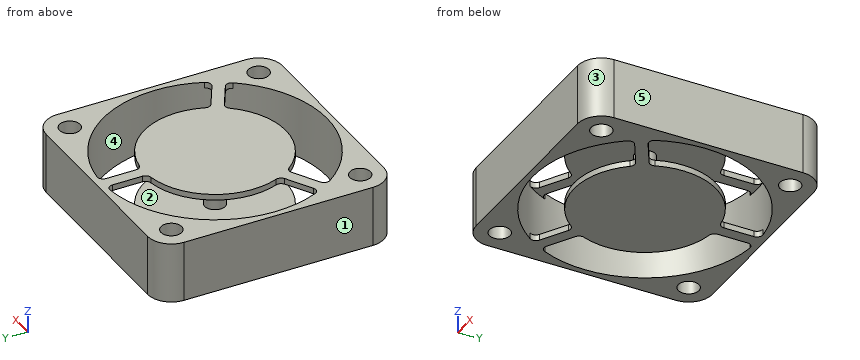
from build123d import *

# Parameters (mm, degrees)
BOSS_EXTRUDE1_DEPTH = 10.3
SKETCH2_R           = 1.75
CUT_EXTRUDE1_DEPTH  = 11.3
SKETCH3_R           = 19
SKETCH3_R_2         = 12
CUT_EXTRUDE2_DEPTH  = 11.3
BOSS_EXTRUDE2_DEPTH = 10.3
CIRPATTERN1_COUNT   = 3
FILLET2_R           = 1
CUT_EXTRUDE3_START  = 1
SKETCH5_R           = 19
CUT_EXTRUDE3_DEPTH  = 8.3
SKETCH6_R           = 1.75
BOSS_EXTRUDE3_DEPTH = 8.3


with BuildPart() as part:
    # Sketch1 → Boss-Extrude1 (new body)
    with BuildSketch(Plane.XY):
        with BuildLine():
            Line((0, -4), (32, -4))
            ThreePointArc((32, -4), (34.828427125, -2.828427125), (36, 0))
            Line((36, 0), (36, 32))
            ThreePointArc((36, 32), (34.828427125, 34.828427125), (32, 36))
            Line((32, 36), (0, 36))
            ThreePointArc((0, 36), (-2.828427125, 34.828427125), (-4, 32))
            Line((-4, 32), (-4, 0))
            ThreePointArc((-4, 0), (-2.828427125, -2.828427125), (0, -4))
        make_face()
    extrude(amount=BOSS_EXTRUDE1_DEPTH)

    # Sketch2 → Cut-Extrude1 (cut, through all)
    with BuildSketch(Plane.XY.offset(10.3)):
        Circle(SKETCH2_R)
        with Locations((0, 32)):
            Circle(SKETCH2_R)
        with Locations((32, 0)):
            Circle(SKETCH2_R)
        with Locations((32, 32)):
            Circle(SKETCH2_R)
    extrude(amount=-CUT_EXTRUDE1_DEPTH, mode=Mode.SUBTRACT)

    # Sketch3 → Cut-Extrude2 (cut, through all)
    with BuildSketch(Plane.XY.offset(10.3)):
        with Locations((16, 16)):
            Circle(SKETCH3_R)
        with Locations((16, 16)):
            Circle(SKETCH3_R_2, mode=Mode.SUBTRACT)
    extrude(amount=-CUT_EXTRUDE2_DEPTH, mode=Mode.SUBTRACT)

    # Sketch4 → Boss-Extrude2 (add)
    with BuildSketch(Plane.XY):
        with BuildLine():
            Line((15, 27.958260743), (15, 34.973665961))
            ThreePointArc((15, 34.973665961), (16, 35), (17, 34.973665961))
            Line((17, 34.973665961), (17, 27.958260743))
            ThreePointArc((17, 27.958260743), (16, 28), (15, 27.958260743))
        make_face()
    boss_extrude2 = extrude(amount=BOSS_EXTRUDE2_DEPTH)

    # CirPattern1: Boss-Extrude2 ×3 about axis
    cirpattern1_axis = Axis((16, 16, 0), (0, 0, 1))
    for i in range(1, CIRPATTERN1_COUNT):
        add(boss_extrude2.rotate(cirpattern1_axis, i * 360 / CIRPATTERN1_COUNT))

    # Fillet2
    fillet2_edges = [part.edges().sort_by_distance(p)[0] for p in [
        (15, 27.958260743, 5.15),
        (17, 27.958260743, 5.15),
        (17, 34.973665961, 5.15),
        (15, 34.973665961, 5.15),
        (6.143842411, 9.154844225, 5.15),
        (5.143842411, 10.886895032, 5.15),
        (-0.931676725, 7.379192423, 5.15),
        (0.068323275, 5.647141616, 5.15),
        (26.856157589, 10.886895032, 5.15),
        (25.856157589, 9.154844225, 5.15),
        (31.931676725, 5.647141616, 5.15),
        (32.931676725, 7.379192423, 5.15),
    ]]
    fillet(fillet2_edges, radius=FILLET2_R)

    # Sketch5 → Cut-Extrude3 (cut)
    with BuildSketch(Plane.XY.offset(CUT_EXTRUDE3_START)):
        with Locations((16, 16)):
            Circle(SKETCH5_R)
    extrude(amount=CUT_EXTRUDE3_DEPTH, mode=Mode.SUBTRACT)

    # Sketch6 → Boss-Extrude3 (add)
    with BuildSketch(Plane.XY.offset(1)):
        with Locations((16, 16)):
            Circle(SKETCH6_R)
    extrude(amount=BOSS_EXTRUDE3_DEPTH)


solid = part.part
Geometry check sheet. Reference: the model listing, model coordinates, mm. Face numbers are marked on the shaded views. A direction names the side the tool comes from. Give positions to 0.01 mm unless a question says otherwise; leave off trailing zeros. Write each loop counter-clockwise with the first axis right and the second up, starting at its lowest first coordinate (ties: lowest second). Pieces come first, ordered by that corner, then holes. Notation, with made-up numbers: M -19,53.25 L 16,53.25 A19 cw 16,73.25 Z; hole C -34,-38.75 d5. An arc over 180 degrees is marked long. Answer as CSV lines item,"result". Start each with the question number.
Q1. Section check C-C, the plane y = 19.5. Record the cut outline in (x, z), then the cut area to 3 significant figures.
Q2. Section check A-A, the plane x = 16. Record the cut outline in (y, z).
Q3. Section check D-D, the plane x = 28.5. Record the cut outline in (y, z).
Q4. Section check B-B, the plane z = 3.5. Record the cut outline in (x, y), then the cut area to 3 significant figures.
Q5. Tool access check on the marked faces 1 and 2. Record the directions out of +Z, -Z, +X, -X, +Y, -Y that give a thin tool (end or side, any length) a straight path to the whole face; none if there is none.
Q6. Release check for a two-part mould opening along Y. For the marked faces 3, 4 and 5 record: pulls with the +Y half, pulls with the -Y half, needs draft (parallel to the pull), parting line crosses it, or undercut.
Q7. Go/stop test with a flat-tipped pin: pin 1 (4 mm diameter, centred on x = 32, y = 0, fed in from -Z). Record where the tip stops, or that it passes through.
Q8. Material ranges on L1, parallel to X at y = 27, z = 3; L2, parallel to X at y = 1.5, z = 2; L3, parallel to Y at x = 0, z = 4.5, recorded low to high.
Geometry says:
1,outline,"M -4,0 L -2.67,0 L -2.67,10.3 L -4,10.3 Z; M 4.52,0 L 27.48,0 L 27.48,1 L 4.52,1 Z; M 4.52,9.3 L 27.48,9.3 L 27.48,10.3 L 4.52,10.3 Z; M 34.67,0 L 36,0 L 36,10.3 L 34.67,10.3 Z"
1,area,"73.2 mm^2"
2,outline,"M -4,0 L -3,0 L -3,10.3 L -4,10.3 Z; M 4,0 L 36,0 L 36,10.3 L 4,10.3 L 4,9.3 L 14.25,9.3 L 14.25,1 L 4,1 Z; hole M 17.75,1 L 35,1 L 35,9.3 L 17.75,9.3 Z"
3,outline,"M -4,0 L 1.69,0 L 1.69,10.3 L -4,10.3 Z; M 7.63,0 L 9.94,0 L 9.94,1 L 7.63,1 Z; M 7.63,9.3 L 9.94,9.3 L 9.94,10.3 L 7.63,10.3 Z; M 30.31,0 L 36,0 L 36,10.3 L 30.31,10.3 Z"
4,outline,"M -4,0 A4 ccw 0,-4 L 32,-4 A4 ccw 36,0 L 36,32 A4 ccw 32,36 L 0,36 A4 ccw -4,32 Z; C 16,16 d3.5; hole C 16,16 d38; hole C 0,0 d3.5; hole C 0,32 d3.5; hole C 32,0 d3.5; hole C 32,32 d3.5"
4,area,"423 mm^2"
5,face 1,"+Z, -Z, -X, +Y, -Y"
5,face 2,"none"
6,face 3,"pulls with the -Y half"
6,face 4,"undercut"
6,face 5,"needs draft"
7,pin 1,"z = 0"
8,L1,"-4 to 0.51, 31.49 to 36"
8,L2,"-4 to -0.9, 0.9 to 3.72, 28.28 to 31.1, 32.9 to 36"
8,L3,"-4 to -1.75, 1.75 to 5.75, 26.25 to 30.25, 33.75 to 36"
